Design review of the part built by this model. Coordinates are the model's own, in mm. A direction names the side the tool comes from. Give positions to 0.01 mm unless a question says otherwise; leave off trailing zeros. Order: outer loops, then holes, each group sorted by start corner. A loop starts at its lowest first (then second) coordinate and runs counter-clockwise, first axis right, second up. Notation, with made-up numbers: (-18, 16.5) -> (18, 16.5) arc R21 ccw to (18, 22.5) -> close; hole circle Ø10 at (62, -26.75). An arc over 180 degrees is marked (long way). Return JSON: item names as keys, results as strings.
```python
from build123d import *
from build123d.topology import SkipClean

# Parameters (mm, degrees)
BOSS_EXTRUDE1_DEPTH = 1.5875
SKETCH2_R           = 6.35
BOSS_EXTRUDE2_DEPTH = 0.79375
FILLET1_R           = 0.5


with BuildPart() as part:
    # Sketch1 → Boss-Extrude1 (new body)
    with BuildSketch(Plane.XY):
        with BuildLine():
            Line((-1.5875, 3.175), (-1.5875, 1.5875))
            Line((-1.5875, 1.5875), (-3.175, 1.5875))
            Line((-3.175, 1.5875), (-3.175, -1.5875))
            Line((-3.175, -1.5875), (-1.5875, -1.5875))
            Line((-1.5875, -1.5875), (-1.5875, -3.175))
            Line((-1.5875, -3.175), (1.5875, -3.175))
            Line((1.5875, -3.175), (1.5875, -1.5875))
            Line((1.5875, -1.5875), (3.175, -1.5875))
            Line((3.175, -1.5875), (3.175, 1.5875))
            Line((3.175, 1.5875), (1.5875, 1.5875))
            Line((1.5875, 1.5875), (1.5875, 3.175))
            Line((1.5875, 3.175), (5.499261314, 3.175))
            ThreePointArc((5.499261314, 3.175), (0, -6.35), (-5.499261314, 3.175))
            Line((-5.499261314, 3.175), (-1.5875, 3.175))
        make_face()
    extrude(amount=BOSS_EXTRUDE1_DEPTH)

    # Sketch2 → Boss-Extrude2 (add)
    with SkipClean():  # the faces are left unmerged after this step: merging them gives an invalid solid
        with BuildSketch(Plane.XY.offset(1.5875)):
            with Locations(Location((0, 0, 0), (0, 0, 150))):
                Circle(SKETCH2_R)
        extrude(amount=BOSS_EXTRUDE2_DEPTH)

    # Fillet1
    fillet1_edges = [part.edges().sort_by_distance(p)[0] for p in [
        (-1.5875, 1.5875, 0.79375),
        (-1.5875, -1.5875, 0.79375),
        (1.5875, -1.5875, 0.79375),
        (1.5875, 1.5875, 0.79375),
    ]]
    fillet(fillet1_edges, radius=FILLET1_R)


solid = part.part
```
Item 1: For pin 1 (1.2 mm diameter, centred on x = -2.5, z = 0.5, fed in from +Y) (3 decimals); pin 2 (0.9 mm diameter, centred on x = -2.5, z = 0.5, fed in from -Y); pin 3 (0.9 mm diameter, centred on y = 2.5, z = 1, fed in from +X), all flat-tipped, find the tip position at first contact; note any pin that passes through.
Result set:
{"pin 1": "stops at y = 3.175", "pin 2": "stops at y = -6.01", "pin 3": "stops at x = 6.01"}
Item 2: Machinability: for faces 3 (the face through (0, -4, 0)), 4 (the face through (-3.175, 0, 1)), 5 (the face through (-4, 3.175, 1)), 6 (the face through (1.588, -3, 1)), which of the approach directions +Z, -Z, +X, -X, +Y, -Y give a long, thin tool a straight path to every point of the face, cutting with its end or side? Answer none if there is none.
Result set:
{"face 3": "-Z, +X, -X, +Y, -Y", "face 4": "-Z", "face 5": "-Z, +X, -X, +Y", "face 6": "-Z, +Y"}
Item 3: Mouldability with a two-part tool opening along X and no side actions: class faces 1 (the face through (0, -3.175, 1)), 2 (the face through (4, 3.175, 1)) as released by +X, released by -X, zero draft, split by the parting line, or undercut.
Result set:
{"face 1": "undercut", "face 2": "zero draft"}
Item 4: Add section D-D (y = -2.75). Give the boundary of the cut face in (x, z), plus the area to 3 significant figures.
Result set:
{"outline": "(-5.72, 0) -> (-1.59, 0) -> (-1.59, 1.59) -> (1.59, 1.59) -> (1.59, 0) -> (5.72, 0) -> (5.72, 2.38) -> (-5.72, 2.38) -> close", "area": "22.2 mm^2"}
Item 5: Wall thickness on L1, parallel to X at y = 0, z = 0.25 (3 decimals); L2, parallel to X at y = 2.25, z = 1.5; L3, parallel to Y at x = -2.25, z = 0.6 (1 decimal): over which ranges is each line inside the solid? List them lowest first. Write a range as [from, to].
Result set:
{"L1": "x = [-6.35, -3.175], [3.175, 6.35]", "L2": "x = [-5.94, -1.59], [1.59, 5.94]", "L3": "y = [-5.9, -1.6], [1.6, 3.2]"}
